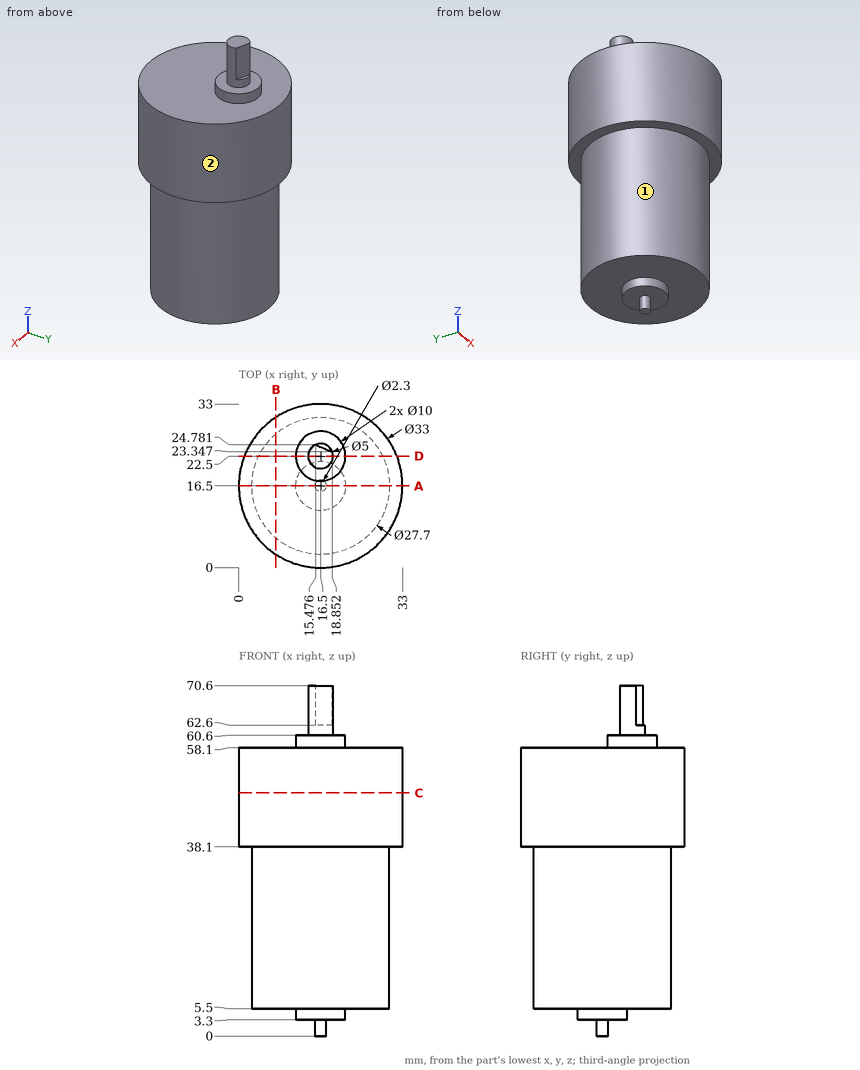
Print and shaded views of the part. All mm, measured from the part's lowest x, y and z. A direction names the side the tool comes from. Give positions to 0.01 mm unless a question says otherwise; leave off trailing zeros. Order: outer loops, then holes, each group sorted by start corner. A loop starts at its lowest first (then second) coordinate and runs counter-clockwise, first axis right, second up. Notation, with made-up numbers: M 42.5,54 L 87.5,54 A21 ccw 87.5,88 Z; hole C -17.75,83.5 d4. An arc over 180 degrees is marked long. Use one line per item in the form item = value.
Q1. Slice it at D-D, the plane y = 22.5. Write the cut outline in (x, z), and give its area (3 significant figures).
Conclusion:
outline = M 1.13,38.1 L 4.02,38.1 L 4.02,5.5 L 28.98,5.5 L 28.98,38.1 L 31.87,38.1 L 31.87,58.1 L 21.5,58.1 L 21.5,60.6 L 19,60.6 L 19,70.6 L 14,70.6 L 14,60.6 L 11.5,60.6 L 11.5,58.1 L 1.13,58.1 Z
area = 1,500 mm2
Q2. Slice it at C-C, the plane z = 49. Write the cut outline in (x, y), and give its area (3 significant figures).
Conclusion:
outline = C 16.5,16.5 d33
area = 855 mm2
Q3. Wall check: probe 1 along Z at (x, y) = (24.5, 6.5); probe 2 along Y at (x, z) = (16, 36); probe 3 along Z at (x, y) = (1.5, 23). Give the ranges that are in metal, low to high.
Conclusion:
probe_1 = 5.5 to 58.1
probe_2 = 2.66 to 30.34
probe_3 = 38.1 to 58.1
Q4. Which spindle directions (+Z, -Z, +X, -X, +Y, -Y) get a long thin tool onto all of the face, cutting with end or side? Do the marked faces 1 and 2. Say none if no direction does.
Conclusion:
face_1 = -Z
face_2 = +Z, -Z
Q5. Slice it at B-B, the plane x = 7.5. Write the cut outline in (y, z), and give its area (3 significant figures).
Conclusion:
outline = M 2.67,38.1 L 5.97,38.1 L 5.97,5.5 L 27.03,5.5 L 27.03,38.1 L 30.33,38.1 L 30.33,58.1 L 2.67,58.1 Z
area = 1,240 mm2
Q6. Pin check, flat tips, straight feed: P1, Ø8, axis at y = 19, z = 21, coming from the +X side; P2, Ø3, axis at y = 12, z = 15.5, coming from the -X side; P3, Ø3, axis at x = 28, y = 7, coming from the +Z side. Stop position of each tip, or through.
Conclusion:
P1 = 30.35
P2 = 2.98
P3 = 58.1
Q7. Slice it at A-A, the plane y = 16.5. Write the cut outline in (x, z), and give its area (3 significant figures).
Conclusion:
outline = M 0,38.1 L 2.65,38.1 L 2.65,5.5 L 11.5,5.5 L 11.5,3.3 L 15.35,3.3 L 15.35,0 L 17.65,0 L 17.65,3.3 L 21.5,3.3 L 21.5,5.5 L 30.35,5.5 L 30.35,38.1 L 33,38.1 L 33,58.1 L 0,58.1 Z
area = 1,590 mm2
